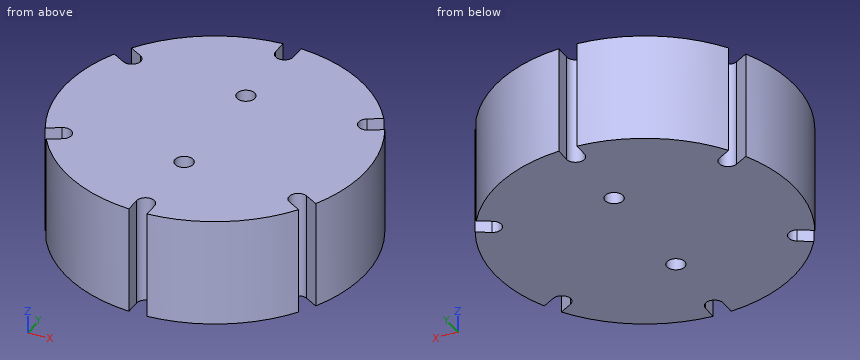
```python
from build123d import *

# Parameters (mm, degrees)
F0_R     = 7.5
F1_DEPTH = 90


with BuildPart() as f1:
    # F0 (on Top) → F1 (new body)
    with BuildSketch(Plane.XY):
        with BuildLine():
            Line((-7.5, 112.5), (-7.5, 124.774797))
            ThreePointArc((-7.5, 124.774797), (-62.5, 108.253175), (-104.308144, 68.882589))
            Line((-104.308144, 68.882589), (-93.677858, 62.745191))
            ThreePointArc((-93.677858, 62.745191), (-90.932667, 52.5), (-101.177858, 49.754809))
            Line((-101.177858, 49.754809), (-111.808144, 55.892208))
            ThreePointArc((-111.808144, 55.892208), (-125, 0), (-111.808144, -55.892208))
            Line((-111.808144, -55.892208), (-101.177858, -49.754809))
            ThreePointArc((-101.177858, -49.754809), (-90.932667, -52.5), (-93.677858, -62.745191))
            Line((-93.677858, -62.745191), (-104.308144, -68.882589))
            ThreePointArc((-104.308144, -68.882589), (-62.5, -108.253175), (-7.5, -124.774797))
            Line((-7.5, -124.774797), (-7.5, -112.5))
            ThreePointArc((-7.5, -112.5), (0, -105), (7.5, -112.5))
            Line((7.5, -112.5), (7.5, -124.774797))
            ThreePointArc((7.5, -124.774797), (62.5, -108.253175), (104.308144, -68.882589))
            Line((104.308144, -68.882589), (93.677858, -62.745191))
            ThreePointArc((93.677858, -62.745191), (90.932667, -52.5), (101.177858, -49.754809))
            Line((101.177858, -49.754809), (111.808144, -55.892208))
            ThreePointArc((111.808144, -55.892208), (125, 0), (111.808144, 55.892208))
            Line((111.808144, 55.892208), (101.177858, 49.754809))
            ThreePointArc((101.177858, 49.754809), (90.932667, 52.5), (93.677858, 62.745191))
            Line((93.677858, 62.745191), (104.308144, 68.882589))
            ThreePointArc((104.308144, 68.882589), (62.5, 108.253175), (7.5, 124.774797))
            Line((7.5, 124.774797), (7.5, 112.5))
            ThreePointArc((7.5, 112.5), (0, 105), (-7.5, 112.5))
        make_face()
        with Locations((0, -50)):
            Circle(F0_R, mode=Mode.SUBTRACT)
        with Locations((0, 50)):
            Circle(F0_R, mode=Mode.SUBTRACT)
    extrude(amount=F1_DEPTH)


with BuildPart() as f1_1:
    # F2: moved
    add(f1.part.moved(Location((0, 0, -90))))


solid = f1_1.part
```
Check sheet for the modelled part. Datum: model origin and axes. Units: mm. Give positions to 0.01 mm unless a question says otherwise; leave off trailing zeros. Write each loop counter-clockwise with the first axis right and the second up, starting at its lowest first coordinate (ties: lowest second). Pieces come first, ordered by that corner, then holes. Notation, with made-up numbers: (58, -37) -> (87, -37) arc R26 ccw to (87, -7) -> close; hole circle Ø5 at (-18, 57). An arc over 180 degrees is marked (long way). Use CSV: the item, a comma, the result in double quotes. Start each with the question number.
Q1. Cross-section at C-C on y = 74.5. Enter the section's corners in (x, z), and give its area (3 significant figures).
Q2. Cross-section at A-A on z = -62. Enter the section's corners in (x, y), and give its area (3 significant figures).
Q3. Cross-section at B-B on x = -25.5. Enter the section's corners in (y, z), and give its area (3 significant figures).
Q4. Depth check by flat-ended pin: P1, Ø10, axis at y = 21, z = -47, coming from the +X side; P2, Ø5, axis at y = -30, z = -15.5, coming from the -X side; P3, Ø13.5, axis at y = -118.5, z = -67, coming from the +X side. Enter the tip coordinate at first touch or a pass-through.
Q5. Scan lines: line 1 along Y through (x, z) = (0, -48.5); line 2 along X through (y, z) = (-54, -54); line 3 along X through (y, z) = (8.5, -58). Record each from-to range of solid material in increasing order.
Working result:
1,outline,"(-100.37, -90) -> (100.37, -90) -> (100.37, 0) -> (-100.37, 0) -> close"
1,area,"18,100 mm^2"
2,outline,"(-111.81, -55.89) -> (-101.18, -49.75) arc R7.5 cw to (-93.68, -62.75) -> (-104.31, -68.88) arc R125 ccw to (-7.5, -124.77) -> (-7.5, -112.5) arc R7.5 cw to (7.5, -112.5) -> (7.5, -124.77) arc R125 ccw to (104.31, -68.88) -> (93.68, -62.75) arc R7.5 cw to (101.18, -49.75) -> (111.81, -55.89) arc R125 ccw to (111.81, 55.89) -> (101.18, 49.75) arc R7.5 cw to (93.68, 62.75) -> (104.31, 68.88) arc R125 ccw to (7.5, 124.77) -> (7.5, 112.5) arc R7.5 cw to (-7.5, 112.5) -> (-7.5, 124.77) arc R125 ccw to (-104.31, 68.88) -> (-93.68, 62.75) arc R7.5 cw to (-101.18, 49.75) -> (-111.81, 55.89) arc R125 ccw to start; hole circle Ø15 at (0, -50); hole circle Ø15 at (0, 50)"
2,area,"47,100 mm^2"
3,outline,"(-122.37, -90) -> (122.37, -90) -> (122.37, 0) -> (-122.37, 0) -> close"
3,area,"22,000 mm^2"
4,P1,"stops at x = 123.97"
4,P2,"stops at x = -121.94"
4,P3,"stops at x = 56.01"
5,line 1,"y = -105 to -57.5, -42.5 to 42.5, 57.5 to 105"
5,line 2,"x = -112.73 to -108.53, -90.27 to -6.34, 6.34 to 90.27, 108.53 to 112.73"
5,line 3,"x = -124.71 to 124.71"
